The figure shows three views and two pictorial views of one solid part (mm, origin at its lowest corner). Answer the questions. Round coordinates to 2 decimals unless told otherwise and drop trailing zeros. Order: outer loops, then holes, each group sorted by start corner. A loop starts at its lowest first (then second) coordinate and runs counter-clockwise, first axis right, second up. Notation, with made-up numbers: M 71.25,-36.5 L 79.25,-36.5 A30 ccw 79.25,1.5 Z; hole C 86,18 d8. An arc over 180 degrees is marked long. Answer as CSV lines item,"result".
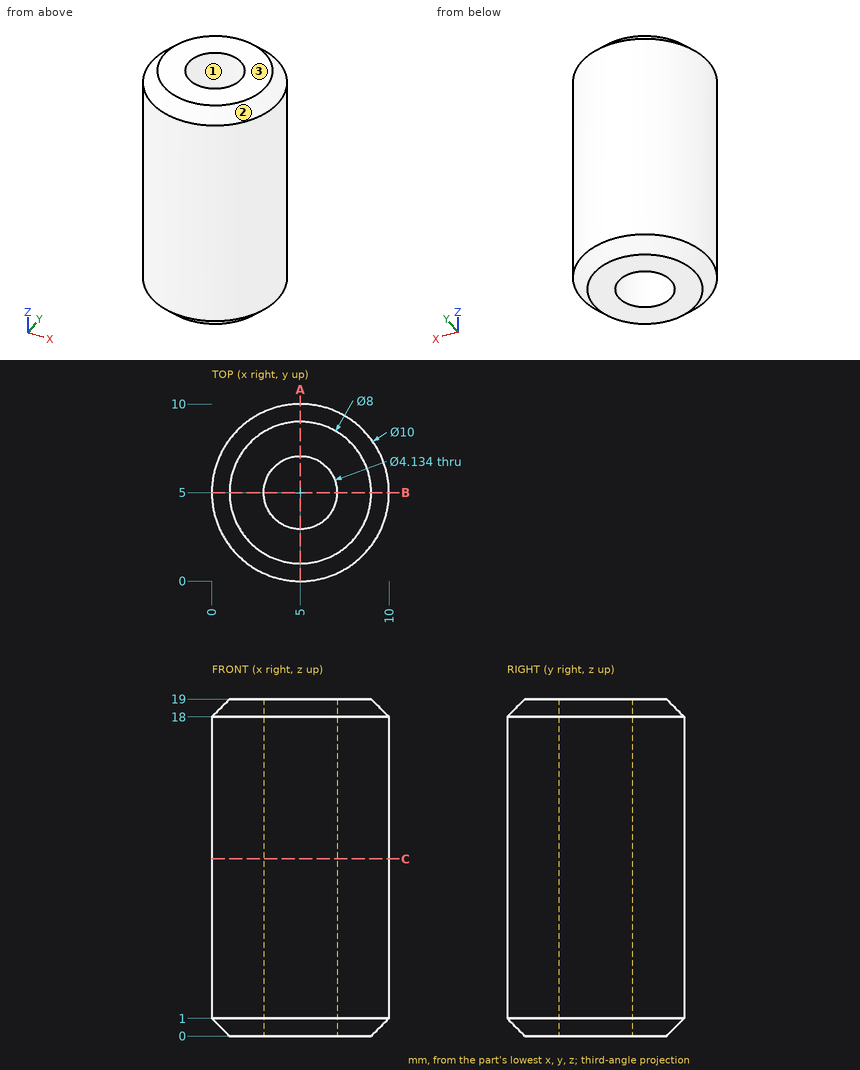
Item 1: Find the intervals of material crossed by probe 1 along Y at (x, z) = (5, 8.5); probe 2 along Y at (x, z) = (5.5, 6.5); probe 3 along X at (y, z) = (6, 7.25), in increasing order. Write a range as [from, to].
Ans:
probe 1,"[0, 2.93], [7.07, 10]"
probe 2,"[0.03, 2.99], [7.01, 9.97]"
probe 3,"[0.1, 3.19], [6.81, 9.9]"
Item 2: Flat-ended cylindrical pins translate along their axes: pin 1 (4 mm diameter, centred on y = 9, z = 14, fed in from +X); pin 2 (2 mm diameter, centred on x = 3.5, z = 15, fed in from -Y); pin 3 (3.5 mm diameter, centred on x = 5, y = 5, fed in from +Z); pin 4 (3 mm diameter, centred on y = 2.5, z = 11.5, fed in from +X). Find the tip coordinate at first contact, or state that the pin passes through.
Ans:
pin 1,"x = 9.58"
pin 2,"y = 0.03"
pin 3,"through"
pin 4,"x = 9.9"
Item 3: A cutting plane is placed at A-A, the plane x = 5. Determine the outline of the cut face in (y, z), and give its area (3 significant figures).
Ans:
outline,"M 0,1 L 1,0 L 2.93,0 L 2.93,19 L 1,19 L 0,18 Z; M 7.07,0 L 9,0 L 10,1 L 10,18 L 9,19 L 7.07,19 Z"
area,"109 mm2"
Item 4: Determine the mould class of the marked faces 1, 2 and 3 for opening direction X: +X half, -X half, draft (parallel to the pull), parting line (faces both ways), or undercut.
Ans:
face 1,"undercut"
face 2,"parting line"
face 3,"draft"
Item 5: A cutting plane is placed at C-C, the plane z = 10. Determine the outline of the cut face in (x, y), and give its area (3 significant figures).
Ans:
outline,"C 5,5 d10; hole C 5,5 d4.13"
area,"65.1 mm2"
